The drawing under review shows one solid part. Ordinate dimensions are in mm from its lowest x, y, z. Round coordinates to 2 decimals unless told otherwise and drop trailing zeros. Write each loop counter-clockwise with the first axis right and the second up, starting at its lowest first coordinate (ties: lowest second). Pieces come first, ordered by that corner, then holes. Notation, with made-up numbers: (-1, -9) -> (3, -9) arc R14 ccw to (3, -5) -> close; hole circle Ø10 at (58, 71). An arc over 180 degrees is marked (long way). Write item = value, one per line. Start each with the question number.
Item 1: To check wall thickness, follow L1, parallel to Y at x = 10, z = 0.7; L2, parallel to Y at x = 20, z = 1.45; L3, parallel to Y at x = 36, z = 0.6. State the ranges of each line that lie inside material, in increasing order.
Item 2: Add section C-C, the plane y = 30. State the section outline as (x, z) points, then the cut area to 3 significant figures.
Item 3: Add section A-A, the plane x = 20. State the section outline as (y, z) points.
Item 4: Add section B-B, the plane x = 10. State the section outline as (y, z) points.
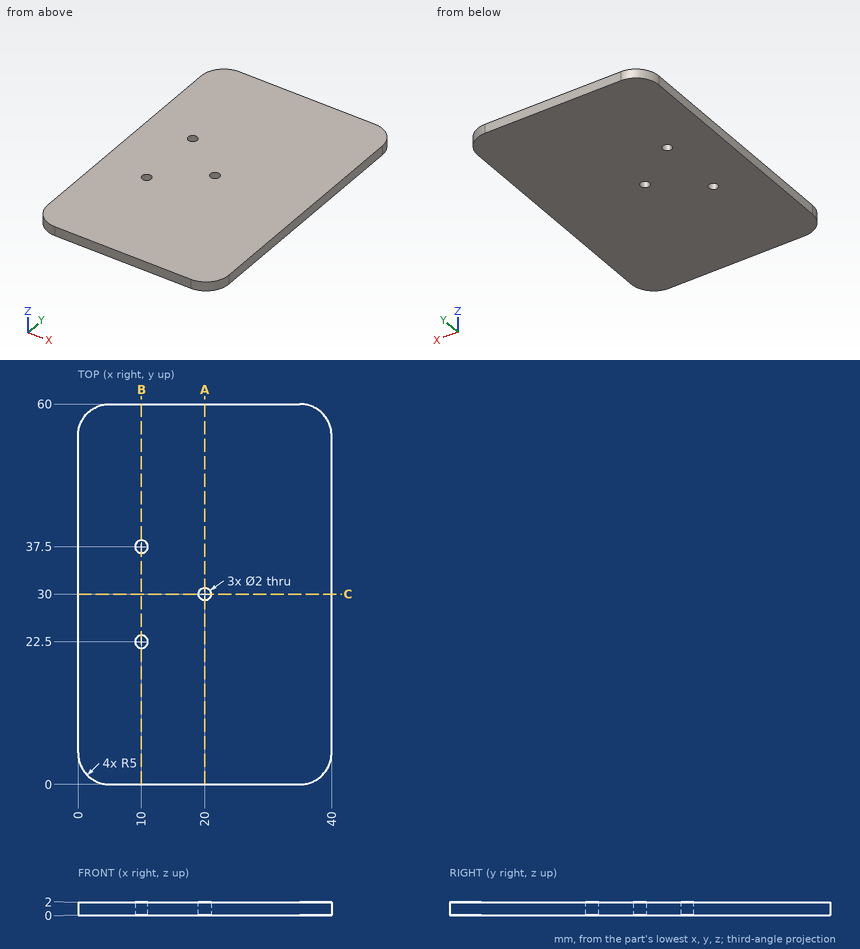
Result set:
q1.L1 = 0 to 21.5, 23.5 to 36.5, 38.5 to 60
q1.L2 = 0 to 29, 31 to 60
q1.L3 = 0.1 to 59.9
q2.outline = (0, 0) -> (19, 0) -> (19, 2) -> (0, 2) -> close; (21, 0) -> (40, 0) -> (40, 2) -> (21, 2) -> close
q2.area = 76.0 mm²
q3.outline = (0, 0) -> (29, 0) -> (29, 2) -> (0, 2) -> close; (31, 0) -> (60, 0) -> (60, 2) -> (31, 2) -> close
q4.outline = (0, 0) -> (21.5, 0) -> (21.5, 2) -> (0, 2) -> close; (23.5, 0) -> (36.5, 0) -> (36.5, 2) -> (23.5, 2) -> close; (38.5, 0) -> (60, 0) -> (60, 2) -> (38.5, 2) -> close
